```python
from build123d import *

# Parameters (mm, degrees)
F1_DEPTH    = 1.5
F2_DEPTH    = 1.5
F3_T1_DEPTH = 28.416407865
F4_R        = 1.25
F5_R        = 1.5
F6_R        = 3


# Not quite as in the source:
# - a fillet or chamfer that OpenCascade refuses, or shapes differently, is made with other operations: its cross-section is extruded or revolved along the edge and cut away or added
# - a feature names something its author has since deleted; it is built from what else it names


with BuildPart() as f1:
    # F0 (on Top) → F1 (new body)
    with BuildSketch(Plane.XY):
        Polygon((40, -35), (40, 35), (-40, 35), (-80, 35), (-70, 30), (-50, -20), (-45, -20), (-40, -35), align=None)
        Polygon((-37.8377223398, -32), (-42.8377223398, -17), (-47.9689011157, -17), (-67.6381773778, 32.1731906551), (-67.2917960675, 32), (-40, 32), (37, 32), (37, -32), align=None, mode=Mode.SUBTRACT)
        Polygon((-47.9689011157, -17), (-42.8377223398, -17), (-37.8377223398, -32), (37, -32), (37, 32), (-40, 32), (-67.2917960675, 32), (-67.6381773778, 32.1731906551), align=None)
    extrude(amount=-F1_DEPTH)

    # F0 (on Top) → F2 (join)
    with BuildSketch(Plane.XY):
        Polygon((40, -35), (40, 35), (-40, 35), (-80, 35), (-70, 30), (-50, -20), (-45, -20), (-40, -35), align=None)
        Polygon((-37.8377223398, -32), (-42.8377223398, -17), (-47.9689011157, -17), (-67.6381773778, 32.1731906551), (-67.2917960675, 32), (-40, 32), (37, 32), (37, -32), align=None, mode=Mode.SUBTRACT)
    extrude(amount=F2_DEPTH)

    # F3: fillet of radius 1.2 on 1 edges, made by hand

    # F3_s2 → F3_t1 (cut)
    with BuildSketch(Plane.XY.offset(-14.2082039325)):
        with BuildLine():
            ThreePointArc((-75.4533747416, 32.7266873708), (-76.0846172144, 34.0757035047), (-74.916718427, 35))
            Line((-74.916718427, 35), (-80, 35))
            Line((-80, 35), (-75.4533747416, 32.7266873708))
        make_face()
    extrude(amount=F3_T1_DEPTH, mode=Mode.SUBTRACT)

    # F4
    f4_edges = [f1.edges().sort_by_distance(p)[0] for p in [
        (-70, 30, 0),
    ]]
    fillet(f4_edges, radius=F4_R)

    # F5
    f5_edges = [f1.edges().sort_by_distance(p)[0] for p in [
        (-45, -20, 0),
        (-40, -35, 0),
    ]]
    fillet(f5_edges, radius=F5_R)

    # F6
    f6_edges = [f1.edges().sort_by_distance(p)[0] for p in [
        (40, -35, 0),
    ]]
    fillet(f6_edges, radius=F6_R)


solid = f1.part
```
Source: CAD feature listing. Evaluate the final solid. Frame: model axes, mm. A direction names the side the tool comes from. Coordinates: 2 decimals unless noted, no trailing zeros. Loops run counter-clockwise (first coordinate to the right, second up) from the corner with the lowest first, then second, coordinate; pieces in that order, holes last. Notation, with made-up numbers: (5.25, -27) - (58.25, -27) arc R32 cw to (58.25, 5) - close; hole circle Ø6 at (27.25, 60.25). An arc over 180 degrees is marked (long way). Answer as CSV lines item,"result".
1. Section C-C (y = -12). Return loops of the section in (x, z).
Established:
outline,"(-53.2, -1.5) - (40, -1.5) - (40, 1.5) - (37, 1.5) - (37, 0) - (-49.97, 0) - (-49.97, 1.5) - (-53.2, 1.5) - close"
2. Mould query, pull axis Y, two halves, no side actions, for faces 4 (the flat face through (-73, 31.5, 0)), 5 (the flat face through (-57.666, 7.242, 0.74)), 6 (the cylindrical face through (-76.09, 34.05, -0.02)). Classes: released by +Y, released by -Y, zero draft, split by the parting line, or undercut.
Established:
face 4,"released by -Y"
face 5,"undercut"
face 6,"split by the parting line"
3. Reachability of faces 1 (the flat face through (-48, -20, 0)), 2 (the flat face through (-40.303, -24.605, 0.74)), 3 (the flat face through (-5, 34, 1.5)) from +Z, -Z, +X, -X, +Y, -Y: full face, straight path, thin tool, end or side. Return the list, or none.
Established:
face 1,"+Z, -Z, -X, -Y"
face 2,"+Z"
face 3,"+Z, +X, -X, +Y, -Y"
4. Section B-B (x = -32.5). Return loops of the section in (y, z), then the cut area to 3 significant figures.
Established:
outline,"(-35, -1.5) - (35, -1.5) - (35, 1.5) - (32, 1.5) - (32, 0) - (-32, 0) - (-32, 1.5) - (-35, 1.5) - close"
area,"114 mm2"
5. Contact query for a flat-ended pin moving along its axis: pin 1 (12 mm diameter, centred on x = 13, y = 23.5, fed in from +Z). Output: stop coordinate, or through.
Established:
pin 1,"stops at z = 0"
6. Ray query, line 1 (Y direction, x = 29.5, z = 1.35); line 2 (X direction, y = 23.5, z = 1.15); line 3 (Z direction, x = 27, y = -13.5). Return the intervals inside material, ascending.
Established:
line 1,"y = -35 to -32, 32 to 35"
line 2,"x = -67.4 to -64.17, 37 to 40"
line 3,"z = -1.5 to 0"
7. Section A-A (z = 0.5). Return loops of the section in (x, y), then the cut area to 3 significant figures.
Established:
outline,"(-75.45, 32.73) - (-70.43, 30.21) arc R1.25 cw to (-69.82, 29.56) - (-50, -20) - (-46.08, -20) arc R1.5 cw to (-44.66, -21.03) - (-40.34, -33.97) arc R1.5 ccw to (-38.92, -35) - (37, -35) arc R3 ccw to (40, -32) - (40, 35) - (-74.92, 35) arc R1.2 ccw to start; hole (-67.64, 32.17) - (-47.97, -17) - (-42.84, -17) - (-37.84, -32) - (37, -32) - (37, 32) - (-67.29, 32) - close"
area,"1,000 mm2"
